from build123d import *

# Parameters (mm, degrees)
SKETCH1_W               = 20
SKETCH1_H               = 20
BOSS_EXTRUDE1_DEPTH     = 30
SKETCH2_R               = 1
CUT_EXTRUDE1_DEPTH      = 2.5
SKETCH3_R               = 8
BOSS_EXTRUDE2_DEPTH     = 1.5
SKETCH4_R               = 2
BOSS_EXTRUDE3_DEPTH     = 10
CUT_EXTRUDE2_DEPTH      = 11
CUT_EXTRUDE2_DEPTH_BACK = 11
CHAMFER1_SIZE           = 0.25
FILLET1_R               = 1
SKETCH6_W               = 10
SKETCH6_H               = 2.5
BOSS_EXTRUDE4_DEPTH     = 12


with BuildPart() as part:
    # Sketch1 → Boss-Extrude1 (new body)
    with BuildSketch(Plane(origin=(0, 0, 0), x_dir=(1, 0, 0), z_dir=(0, 1, 0))):
        Rectangle(SKETCH1_W, SKETCH1_H)
    extrude(amount=-BOSS_EXTRUDE1_DEPTH)

    # Sketch2 → Cut-Extrude1 (cut)
    with BuildSketch(Plane(origin=(0, 0, 0), x_dir=(1, 0, 0), z_dir=(0, 1, 0))):
        with Locations((-7.7, 7.7)):
            Circle(SKETCH2_R)
        with Locations((7.7, 7.7)):
            Circle(SKETCH2_R)
        with Locations((7.7, -7.7)):
            Circle(SKETCH2_R)
        with Locations((-7.7, -7.7)):
            Circle(SKETCH2_R)
    extrude(amount=-CUT_EXTRUDE1_DEPTH, mode=Mode.SUBTRACT)

    # Sketch3 → Boss-Extrude2 (add)
    with BuildSketch(Plane(origin=(0, 0, 0), x_dir=(1, 0, 0), z_dir=(0, 1, 0))):
        Circle(SKETCH3_R)
    extrude(amount=BOSS_EXTRUDE2_DEPTH)

    # Sketch4 → Boss-Extrude3 (add)
    with BuildSketch(Plane(origin=(0, 0, 0), x_dir=(1, 0, 0), z_dir=(0, 1, 0))):
        Circle(SKETCH4_R)
    extrude(amount=BOSS_EXTRUDE3_DEPTH)

    # Sketch5 → Cut-Extrude2 (cut, two sides)
    with BuildSketch(Plane.XY) as cut_extrude2_sk:
        Polygon((2, 10), (1.5, 10), (1.5, 3), (2, 2.5), align=None)
    extrude(amount=CUT_EXTRUDE2_DEPTH, mode=Mode.SUBTRACT)
    extrude(cut_extrude2_sk.sketch, amount=-CUT_EXTRUDE2_DEPTH_BACK, mode=Mode.SUBTRACT)

    # Chamfer1
    chamfer1_edges = [part.edges().sort_by_distance(p)[0] for p in [
        (-2, 10, 0),
    ]]
    chamfer(chamfer1_edges, length=CHAMFER1_SIZE)

    # Fillet1
    fillet1_edges = [part.edges().sort_by_distance(p)[0] for p in [
        (10, -30, 0),
        (0, -30, -10),
        (-10, -30, 0),
        (0, -30, 10),
        (-10, -15, -10),
        (10, -15, -10),
        (10, -15, 10),
        (-10, -15, 10),
    ]]
    fillet(fillet1_edges, radius=FILLET1_R)

    # Sketch6 → Boss-Extrude4 (add)
    with BuildSketch(Plane(origin=(0, 0, 0), x_dir=(0, 0, -1), z_dir=(1, 0, 0))):
        with Locations((0, -25)):
            Rectangle(SKETCH6_W, SKETCH6_H)
    extrude(amount=BOSS_EXTRUDE4_DEPTH)


solid = part.part
Can you work these out from the model? Positions are in its coordinate system, mm. A direction names the side the tool comes from. Give positions to 0.01 mm unless a question says otherwise; leave off trailing zeros. Order: outer loops, then holes, each group sorted by start corner. A loop starts at its lowest first (then second) coordinate and runs counter-clockwise, first axis right, second up. Notation, with made-up numbers: M 84.25,45 L 130.25,45 A7 cw 130.25,53 Z; hole C -24.5,3.25 d10. An arc over 180 degrees is marked long. Use a Markdown table: item, result. Add a question column.
Item 1: If I drill on L1, parallel to X at y = -1.15, z = -7.7; L2, parallel to X at y = -16, z = -1.25, over which ranges is the centre line in solid material (lowest first)? Write a range as [from, to].
Item 2: For faces 4 (the flat face through (11, -25, 5)), 5 (the flat face through (11, -25, -5)), 6 (the cylindrical face through (-6.776, -1.232, -7.317)), which set-ups out of +Z, -Z, +X, -X, +Y, -Y let a thin tool reach every point of the face, with its end or its side?
Item 3: Suppose I cut it at B-B (y = -23). List the corners of the cut face in (x, z) for me.
Item 4: Suppose I cut it at A-A (z = 0). List the corners of the cut face in (x, y) for me, then the cut area to 3 significant figures.
Item 5: Suppose I cut it at C-C (x = 0). List the corners of the cut face in (y, z) for me, then the cut area to 3 significant figures.
Item 6: Will these pins go through, and if not, where does the flat tip stop? pin 1 (0.6 mm diameter, centred on x = -7.5, z = -7.5, fed in from +Y); pin 2 (0.6 mm diameter, centred on x = 11.5, z = -2.5, fed in from -Y); pin 3 (5.5 mm diameter, centred on y = -19.5, z = -1.5, fed in from +X).
Item 7: Suppose I cut it at D-D (x = 7.5). List the corners of the cut face in (y, z) for me, then the cut area to 3 significant figures.
Item 8: We'd pull the mould along Z, two halves only. Please class faces 1 (the cylindrical face through (8.624, -1.232, -7.317)), 2 (the cylindrical face through (0.126, -29.699, 9.715)), 3 (the flat face through (0, -30, 0)): +Z half, -Z half, draft (parallel to the pull), parting line (faces both ways), or undercut.
Answer sheet:
| question | item | result |
|---|---|---|
| 1 | L1 | x = [-10, -8.7], [-6.7, 6.7], [8.7, 10] |
| 1 | L2 | x = [-10, 10] |
| 2 | face 4 | +Z, +X, +Y, -Y |
| 2 | face 5 | -Z, +X, +Y, -Y |
| 2 | face 6 | +Y |
| 3 | outline | M -10,-9 A1 ccw -9,-10 L 9,-10 A1 ccw 10,-9 L 10,9 A1 ccw 9,10 L -9,10 A1 ccw -10,9 Z |
| 4 | outline | M -10,-29 A1 ccw -9,-30 L 9,-30 A1 ccw 10,-29 L 10,-26.25 L 12,-26.25 L 12,-23.75 L 10,-23.75 L 10,0 L 8,0 L 8,1.5 L 2,1.5 L 2,2.5 L 1.5,3 L 1.5,10 L -1.75,10 L -2,9.75 L -2,1.5 L -8,1.5 L -8,0 L -10,0 Z |
| 4 | area | 659 mm² |
| 5 | outline | M -30,-9 A1 ccw -29,-10 L 0,-10 L 0,-8 L 1.5,-8 L 1.5,-2 L 9.75,-2 L 10,-1.75 L 10,1.75 L 9.75,2 L 1.5,2 L 1.5,8 L 0,8 L 0,10 L -29,10 A1 ccw -30,9 Z |
| 5 | area | 658 mm² |
| 6 | pin 1 | stops at y = -2.5 |
| 6 | pin 2 | stops at y = -26.25 |
| 6 | pin 3 | stops at x = 10 |
| 7 | outline | M -30,-9 A1 ccw -29,-10 L 0,-10 L 0,-8.68 L -2.5,-8.68 L -2.5,-6.72 L 0,-6.72 L 0,-2.78 L 1.5,-2.78 L 1.5,2.78 L 0,2.78 L 0,6.72 L -2.5,6.72 L -2.5,8.68 L 0,8.68 L 0,10 L -29,10 A1 ccw -30,9 Z |
| 7 | area | 598 mm² |
| 8 | face 1 | undercut |
| 8 | face 2 | +Z half |
| 8 | face 3 | draft |
